```python
from build123d import *

# Parameters (mm, degrees)
SKETCH_1_R          = 11.5
SKETCH_1_R_2        = 2.65
EXTRUDE_1_DEPTH     = 2
SKETCH_2_R          = 11.5
EXTRUDE_2_DEPTH     = 1
SKETCH_3_R          = 5
CUT_EXTRUDE_1_DEPTH = 10


with BuildPart() as part:
    # 草图1 → 凸台-拉伸1 (new body)
    with BuildSketch(Plane.XY):
        Circle(SKETCH_1_R)
        with Locations((0, 8)):
            Circle(SKETCH_1_R_2, mode=Mode.SUBTRACT)
        with Locations((8, 0)):
            Circle(SKETCH_1_R_2, mode=Mode.SUBTRACT)
        with Locations(Location((0, -8, 0), (0, 0, 180))):
            Circle(SKETCH_1_R_2, mode=Mode.SUBTRACT)
        with Locations(Location((-8, 0, 0), (0, 0, 180))):
            Circle(SKETCH_1_R_2, mode=Mode.SUBTRACT)
    extrude(amount=EXTRUDE_1_DEPTH)

    # 草图2 → 凸台-拉伸2 (add)
    with BuildSketch(Plane.XY.offset(2)):
        Circle(SKETCH_2_R)
    extrude(amount=EXTRUDE_2_DEPTH)

    # 草图3 → 切除-拉伸1 (cut)
    with BuildSketch(Plane.XY.offset(3)):
        Circle(SKETCH_3_R)
    extrude(amount=-CUT_EXTRUDE_1_DEPTH, mode=Mode.SUBTRACT)


solid = part.part
```
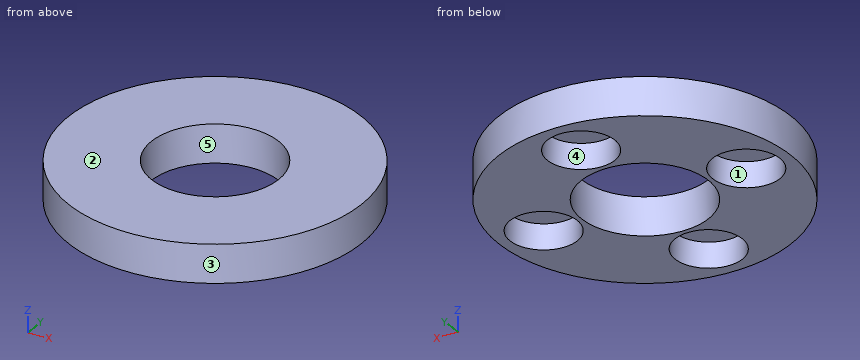
Verification items for the finished model (mm, model axes). Face numbers are marked on the shaded views. A direction names the side the tool comes from. Give positions to 0.01 mm unless a question says otherwise; leave off trailing zeros. Order: outer loops, then holes, each group sorted by start corner. A loop starts at its lowest first (then second) coordinate and runs counter-clockwise, first axis right, second up. Notation, with made-up numbers: M -28.75,-24 L -10.75,-24 A19 cw -10.75,-9 Z; hole C 59,13.5 d5. An arc over 180 degrees is marked long. Answer in a Markdown table with one row per item. Add a question column.
Item 1: Gauge pin test, flat ends, axial feed: pin 1 (5 mm diameter, centred on x = -8, y = 0, fed in from -Z); pin 2 (1.5 mm diameter, centred on y = 8.5, z = 2, fed in from -X). Record the tip position at first contact, or that the pin passes through.
Item 2: Section check D-D, the plane x = -3.5. Enter the section's corners in (y, z), and give its area (3 significant figures).
Item 3: Section check C-C, the plane z = 2.7. Enter the section's corners in (x, y).
Item 4: Tool access check on the marked faces 4 and 5. Record the directions out of +Z, -Z, +X, -X, +Y, -Y that give a thin tool (end or side, any length) a straight path to the whole face; none if there is none.
Item 5: Mould release check, pull along Y, two halves, no side actions. Record for the marked faces 1, 2 and 3: released by +Y, released by -Y, zero draft, split by the parting line, or undercut.
Item 6: Section check A-A, the plane y = 0. Enter the section's corners in (x, z).
Item 7: Scan lines: probe 1 along Y at (x, z) = (0, 1.15); probe 2 along Y at (x, z) = (4.5, 2.75); probe 3 along Z at (x, y) = (-2, 8). Record each from-to range of solid material in increasing order. Write a range as from..to.
Filled sheet:
| question | item | result |
|---|---|---|
| 1 | pin 1 | stops at z = 2 |
| 1 | pin 2 | stops at x = -8.5 |
| 2 | outline | M -10.95,0 L -3.57,0 L -3.57,3 L -10.95,3 Z; M 3.57,0 L 10.95,0 L 10.95,3 L 3.57,3 Z |
| 2 | area | 44.3 mm^2 |
| 3 | outline | C 0,0 d23; hole C 0,0 d10 |
| 4 | face 4 | -Z |
| 4 | face 5 | +Z, -Z |
| 5 | face 1 | undercut |
| 5 | face 2 | zero draft |
| 5 | face 3 | split by the parting line |
| 6 | outline | M -11.5,0 L -10.65,0 L -10.65,2 L -5.35,2 L -5.35,0 L -5,0 L -5,3 L -11.5,3 Z; M 5,0 L 5.35,0 L 5.35,2 L 10.65,2 L 10.65,0 L 11.5,0 L 11.5,3 L 5,3 Z |
| 7 | probe 1 | y = -11.5..-10.65, -5.35..-5, 5..5.35, 10.65..11.5 |
| 7 | probe 2 | y = -10.58..-2.18, 2.18..10.58 |
| 7 | probe 3 | z = 2..3 |
